```python
from build123d import *

# Parameters (mm, degrees)
F0_W      = 55
F0_H      = 30
F1_DEPTH  = 30
F2_W      = 24.7374541685
F2_H      = 14.993442893
F3_DEPTH  = 35
F5_DEPTH  = 5
F7_DEPTH  = 5
F8_R      = 3
F9_W      = 15
F9_H      = 9.6639953554
F10_DEPTH = 33.1
F11_R     = 2
F12_R     = 2.1149349852
F12_R_2   = 1.8799425549
F13_DEPTH = 1
F14_R     = 3
F15_DEPTH = 15
F16_R     = 5
F17_DEPTH = 4
F18_SIZE  = 1.99999


# Not quite as in the source:
# - a fillet or chamfer is up to 0.001 mm smaller than in the source, because OpenCascade refuses the exact size


with BuildPart() as f1:
    # F0 (on Top) → F1 (new body)
    with BuildSketch(Plane.XY):
        with Locations((5.7581346482, 7.7498872403)):
            Rectangle(F0_W, F0_H)
    extrude(amount=F1_DEPTH)

    # F2 (on face) → F3 (cut)
    with BuildSketch(Plane(origin=(0, 22.7498872403, 0), x_dir=(-1, 0, 0), z_dir=(0, 1, 0))):
        with Locations((-20.889407564, 22.5032785535)):
            Rectangle(F2_W, F2_H)
    extrude(amount=-F3_DEPTH, mode=Mode.SUBTRACT)

    # F4 (on face) → F5 (cut)
    with BuildSketch(Plane(origin=(0, 22.7498872403, 0), x_dir=(-1, 0, 0), z_dir=(0, 1, 0))):
        with BuildLine():
            Line((-27.9546213446, 0), (-12.7694251838, 0))
            ThreePointArc((-12.7694251838, 0), (-20.3620232642, 7.5925980804), (-27.9546213446, 0))
        make_face()
        with BuildLine():
            ThreePointArc((17.3747475732, 0), (9.9283689633, 7.4463786099), (2.4819903534, 0))
            Line((2.4819903534, 0), (17.3747475732, 0))
        make_face()
    extrude(amount=-F5_DEPTH, mode=Mode.SUBTRACT)

    # F6 (on face) → F7 (cut)
    with BuildSketch(Plane.XZ.offset(7.2501127597)):
        with BuildLine():
            Line((-16.4975558603, 0), (-1.7069804287, 0))
            ThreePointArc((-1.7069804287, 0), (-9.1022681445, 7.3952877158), (-16.4975558603, 0))
        make_face()
        with BuildLine():
            ThreePointArc((28.6537096156, 0), (20.9127571434, 7.7409524722), (13.1718046712, 0))
            Line((13.1718046712, 0), (28.6537096156, 0))
        make_face()
    extrude(amount=-F7_DEPTH, mode=Mode.SUBTRACT)

    # F8
    f8_edges = [f1.edges().sort_by_distance(p)[0] for p in [
        (8.52068, -7.250113, 22.503279),
        (8.52068, 22.749887, 22.503279),
        (33.258135, 22.749887, 7.503279),
        (33.258135, 7.749887, 15.006557),
        (33.258135, -7.250113, 7.503279),
        (8.52068, 7.749887, 30),
        (-6.610592, 22.749887, 30),
        (-21.741865, 7.749887, 30),
        (20.889408, 22.749887, 15.006557),
        (20.889408, -7.250113, 15.006557),
        (-6.610592, -7.250113, 30),
    ]]
    fillet(f8_edges, radius=F8_R)

    # F9 (on face) → F10 (cut)
    with BuildSketch(Plane.XZ.offset(7.2501127597)):
        with Locations((-11.2023635954, 19.8851507157)):
            Rectangle(F9_W, F9_H)
    extrude(amount=-F10_DEPTH, mode=Mode.SUBTRACT)

    # F11
    f11_edges = [f1.edges().sort_by_distance(p)[0] for p in [
        (-11.202364, 22.749887, 15.053153),
        (-11.202364, -7.250113, 15.053153),
    ]]
    fillet(f11_edges, radius=F11_R)

    # F12 (on face) → F13 (join)
    with BuildSketch(Plane.YZ.offset(33.2581346482)):
        with Locations((-1.053063781, 9.3823140487)):
            Circle(F12_R)
        with Locations((17.056318, 9.5132254064)):
            Circle(F12_R_2)
    extrude(amount=F13_DEPTH)

    # F14 (on face) → F15 (join)
    with BuildSketch(Plane.XY.offset(15.006557107)):
        with Locations((25.5206804797, 8.3661237732)):
            Circle(F14_R)
    extrude(amount=F15_DEPTH)

    # F16 (on face) → F17 (join)
    with BuildSketch(Plane.XY.offset(30.006557107)):
        with Locations((25.5206804797, 8.3661237732)):
            Circle(F16_R)
    extrude(amount=F17_DEPTH)

    # F18 (size 2 in the source; OpenCascade refuses exactly that, so slightly less here)
    f18_edges = [f1.edges().sort_by_distance(p)[0] for p in [
        (20.52068, 8.366124, 30.006557),
    ]]
    chamfer(f18_edges, length=F18_SIZE)


solid = f1.part
```
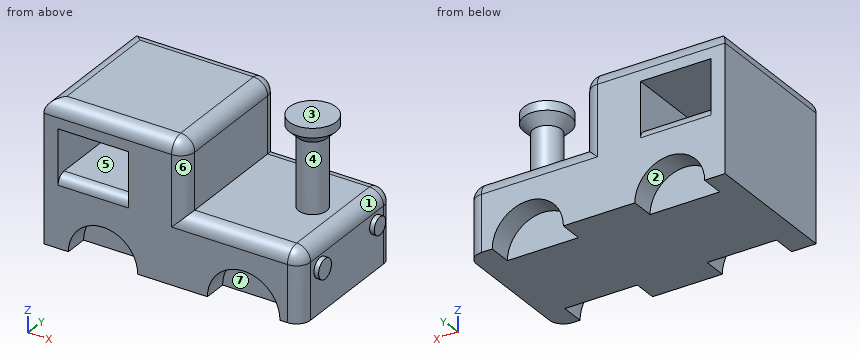
Check sheet for the modelled part. Datum: model origin and axes. Units: mm. Face numbers are marked on the shaded views. A direction names the side the tool comes from. Round coordinates to 2 decimals unless told otherwise and drop trailing zeros. Order: outer loops, then holes, each group sorted by start corner. A loop starts at its lowest first (then second) coordinate and runs counter-clockwise, first axis right, second up. Notation, with made-up numbers: (-14, 61.5) -> (-5, 61.5) arc R22 ccw to (-5, 95.5) -> close; hole circle Ø5 at (8.25, -26.5). An arc over 180 degrees is marked (long way). Use CSV: the item, a comma, the result in double quotes.
(1) Cross-section at D-D (x = 7.5). Record the boundary of the cut face in (y, z).
Worked out:
outline,"(-7.25, 0) -> (22.75, 0) -> (22.75, 12.01) arc R3 ccw to (22, 13.99) -> (22, 27) arc R2.25 ccw to (19.75, 29.25) -> (-4.25, 29.25) arc R2.25 ccw to (-6.5, 27) -> (-6.5, 13.99) arc R3 ccw to (-7.25, 12.01) -> close"
(2) Material ranges on line 1 along X through (y, z) = (6, 18); line 2 along Z through (x, y) = (10.5, 13.5); line 3 along X through (y, z) = (4.25, 24), recorded low to high. Write a range as from..to.
Worked out:
line 1,"-21.74..-18.7, -3.7..8.52, 23.68..27.36"
line 2,"0..15.01"
line 3,"-21.74..-18.7, -3.7..8.52"
(3) Cross-section at A-A (z = 25.5). Record the boundary of the cut face in (x, y), and give its area (3 significant figures).
Worked out:
outline,"(-21.74, -7.25) -> (5.52, -7.25) arc R3 ccw to (8.52, -4.25) -> (8.52, 19.75) arc R3 ccw to (5.52, 22.75) -> (-21.74, 22.75) -> close; circle Ø6 at (25.52, 8.37)"
area,"932 mm²"
(4) Cross-section at C-C (x = -0.5). Record the boundary of the cut face in (y, z), and give its area (3 significant figures).
Worked out:
outline,"(-7.25, 0) -> (22.75, 0) -> (22.75, 27) arc R3 ccw to (19.75, 30) -> (-4.25, 30) arc R3 ccw to (-7.25, 27) -> close"
area,"896 mm²"
(5) Tool access check on the marked faces 5, 6 and 7. Record the directions out of +Z, -Z, +X, -X, +Y, -Y that give a thin tool (end or side, any length) a straight path to the whole face; none if there is none.
Worked out:
face 5,"+Y, -Y"
face 6,"+Z, +X, -Y"
face 7,"-Z, -Y"
(6) Depth check by flat-ended pin: pin 1 (9.5 mm diameter, centred on y = 11, z = 6, fed in from +X); pin 2 (7.5 mm diameter, centred on x = -12.5, y = 5.5, fed in from +Z); pin 3 (4 mm diameter, centred on x = 19, z = 2.5, fed in from +Y). Enter the tip coordinate at first touch or a pass-through.
Worked out:
pin 1,"x = 33.26"
pin 2,"z = 30"
pin 3,"y = 17.75"
(7) Cross-section at B-B (z = 20.5). Record the boundary of the cut face in (x, y).
Worked out:
outline,"(-21.74, -7.25) -> (-18.7, -7.25) -> (-18.7, 22.75) -> (-21.74, 22.75) -> close; (-3.7, -7.25) -> (5.52, -7.25) arc R3 ccw to (8.52, -4.25) -> (8.52, 19.75) arc R3 ccw to (5.52, 22.75) -> (-3.7, 22.75) -> close; circle Ø6 at (25.52, 8.37)"
(8) Draft check along X on the marked faces 1, 2, 3 and 4. Enter one of: pulls with the +X half, pulls with the -X half, needs draft (parallel to the pull), parting line crosses it, or undercut.
Worked out:
face 1,"pulls with the +X half"
face 2,"undercut"
face 3,"needs draft"
face 4,"undercut"
